Source: CAD feature listing. Evaluate the final solid. Frame: model axes, mm. Coordinates: 2 decimals unless noted, no trailing zeros. Loops run counter-clockwise (first coordinate to the right, second up) from the corner with the lowest first, then second, coordinate; pieces in that order, holes last. Notation, with made-up numbers: (67.25, -29.75) -> (91.25, -29.75) arc R33 ccw to (91.25, 2.25) -> close; hole circle Ø2 at (59.5, -22). An arc over 180 degrees is marked (long way). Answer as CSV lines item,"result".
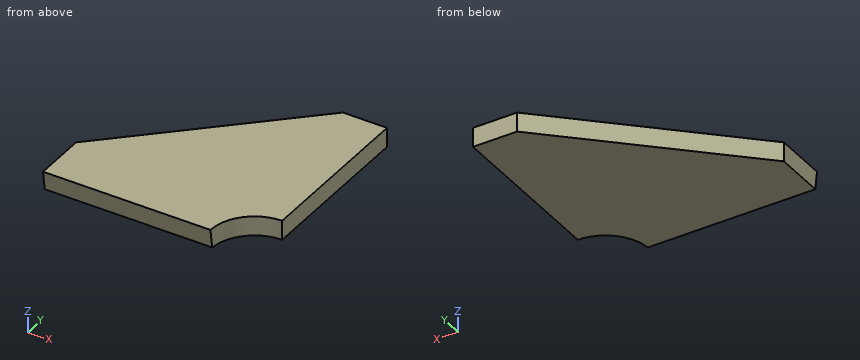
from build123d import *

# Parameters (mm, degrees)
BOSS_EXTRUDE1_DEPTH = 11
CUT_EXTRUDE1_DEPTH  = 114


with BuildPart() as part:
    # Sketch1 → Boss-Extrude1 (new body)
    with BuildSketch(Plane.XY):
        with BuildLine():
            Line((25, 0), (0, 0))
            Line((0, 0), (-95, -90))
            Line((-95, -90), (-95, -120))
            Line((-95, -120), (0, -120))
            ThreePointArc((0, -120), (7.32233047, -102.32233047), (25, -95))
            Line((25, -95), (25, 0))
        make_face()
    extrude(amount=BOSS_EXTRUDE1_DEPTH)

    # Sketch2 → Cut-Extrude1 (cut)
    with BuildSketch(Plane.ZY.offset(95)):
        Polygon((0, -120), (0, -118.454050818), (11, -120), align=None)
    extrude(amount=-CUT_EXTRUDE1_DEPTH, mode=Mode.SUBTRACT)


solid = part.part
(1) Material intervals for L1, parallel to Y at x = -50.5, z = 3.5; L2, parallel to X at y = -63.5, z = 9; L3, parallel to Y at x = -32, z = 6.5, sorted ascending. Write a range as [from, to].
Computed values:
L1,"[-118.95, -47.84]"
L2,"[-67.03, 25]"
L3,"[-119.37, -30.32]"
(2) Cut plane B-B (y = -27). Return the cut outline in (x, z), then the cut area to 4 significant figures.
Computed values:
outline,"(-28.5, 0) -> (25, 0) -> (25, 11) -> (-28.5, 11) -> close"
area,"588.5 mm^2"
(3) Pin query (flat end, axial travel): pin 1 Ø5 at (y, z) = (-88.5, 7) entering from -X; pin 2 Ø1.5 at (x, z) = (-6, 2) entering from -Y; pin 3 Ø6 at (y, z) = (-82, 9.5) entering from -X; pin 4 Ø4 at (x, z) = (-56.5, 2) entering from -Y. Return the tip coordinate at first contact, or that it passes through.
Computed values:
pin 1,"x = -95"
pin 2,"y = -118.84"
pin 3,"x = -89.72"
pin 4,"y = -119.02"
(4) Cut plane C-C (x = -84). Return the cut outline in (y, z).
Computed values:
outline,"(-120, 11) -> (-118.45, 0) -> (-79.58, 0) -> (-79.58, 11) -> close"
(5) Cut plane A-A (z = 4). Return the cut outline in (x, y), then the cut area to 3 significant figures.
Computed values:
outline,"(-95, -119.02) -> (0.02, -119.02) arc R25 cw to (25, -95) -> (25, 0) -> (0, 0) -> (-95, -90) -> close"
area,"9,540 mm^2"
